Here's how the part is built. I have some questions about the finished solid (model axes, mm). Face numbers are marked on the shaded views. A direction names the side the tool comes from. Coordinates: 2 decimals unless noted, no trailing zeros. Write each loop counter-clockwise with the first axis right and the second up, starting at its lowest first coordinate (ties: lowest second). Pieces come first, ordered by that corner, then holes.
```python
from build123d import *

# Parameters (mm, degrees)
SKETCH2_R          = 5
CUT_EXTRUDE1_DEPTH = 50
SKETCH3_R          = 5
CUT_EXTRUDE2_DEPTH = 50


with BuildPart() as part:
    # Sketch1 → Revolve1 (revolve)
    with BuildSketch(Plane.XY):
        with BuildLine():
            Line((238.015458409, 6), (238.015458409, 5))
            Line((238.015458409, 5), (259.308351628, 5))
            Line((259.308351628, 5), (260.015458409, 4.292893219))
            Line((260.015458409, 4.292893219), (260.015458409, 0))
            Line((260.015458409, 0), (-29.984541591, 0))
            Line((-29.984541591, 0), (-29.984541591, 13))
            ThreePointArc((-29.984541591, 13), (-29.105861935, 15.121320344), (-26.984541591, 16))
            Line((-26.984541591, 16), (10.015458409, 16))
            Line((10.015458409, 16), (10.015458409, 9.998359118))
            Line((10.015458409, 9.998359118), (220.015458409, 9.998359118))
            Line((220.015458409, 9.998359118), (220.015458409, 6))
            Line((220.015458409, 6), (238.015458409, 6))
        make_face()
    revolve(axis=Axis((-31.94536444, 0, 0), (1, 0, 0)))

    # Sketch2 → Cut-Extrude1 (cut, symmetric)
    with BuildSketch(Plane(origin=(0, 0, 0), x_dir=(1, 0, 0), z_dir=(0, 1, 0))):
        with Locations((-9.984541591, 0)):
            Circle(SKETCH2_R)
    extrude(amount=CUT_EXTRUDE1_DEPTH, both=True, mode=Mode.SUBTRACT)

    # Sketch3 → Cut-Extrude2 (cut, symmetric)
    with BuildSketch(Plane.XY):
        with Locations((-9.984541591, 0)):
            Circle(SKETCH3_R)
    extrude(amount=CUT_EXTRUDE2_DEPTH, both=True, mode=Mode.SUBTRACT)


solid = part.part
```
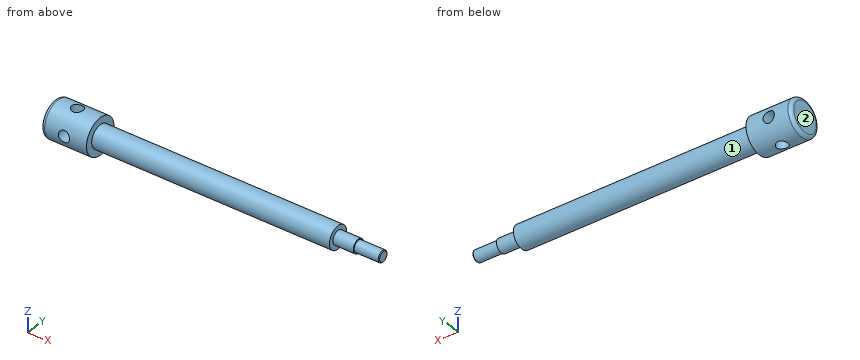
1) Will these pins go through, and if not, where does the flat tip stop? pin 1 (5 mm diameter, centred on x = 173, z = 5.5, fed in from -Y); pin 2 (5 mm diameter, centred on x = 114.5, y = 6.5, fed in from +Z); pin 3 (2 mm diameter, centred on x = 114.5, z = -5, fed in from +Y).
Values follow:
pin 1: stops at y = -9.54
pin 2: stops at z = 9.16
pin 3: stops at y = 9.16
2) I need wall thicknesses on probe 1 along X at (y, z) = (0, 12.5); probe 2 along X at (y, z) = (0, -7); probe 3 along Y at (x, z) = (22, -0.5). Which ranges of each line are inside material? Lowest first, please.
Values follow:
probe 1: x = -29.98 to -14.98, -4.98 to 10.02
probe 2: x = -29.98 to -14.98, -4.98 to 220.02
probe 3: y = -9.99 to 9.99
3) On a 3-axis mill with a long thin cutter (end or side, diameter ignored), from which of +Z, -Z, +X, -X, +Y, -Y can I reach the whole of each face in a straight line? I mean the marked faces 1 and 2. Say none if no direction works.
Values follow:
face 1: +X
face 2: +Z, -Z, -X, +Y, -Y
4) Imagine slicing it at A-A on x = 200. Please give me the cut outline in (y, z), then the cut area to 3 significant figures.
Values follow:
outline: circle Ø20 at (0, 0)
area: 314 mm2
